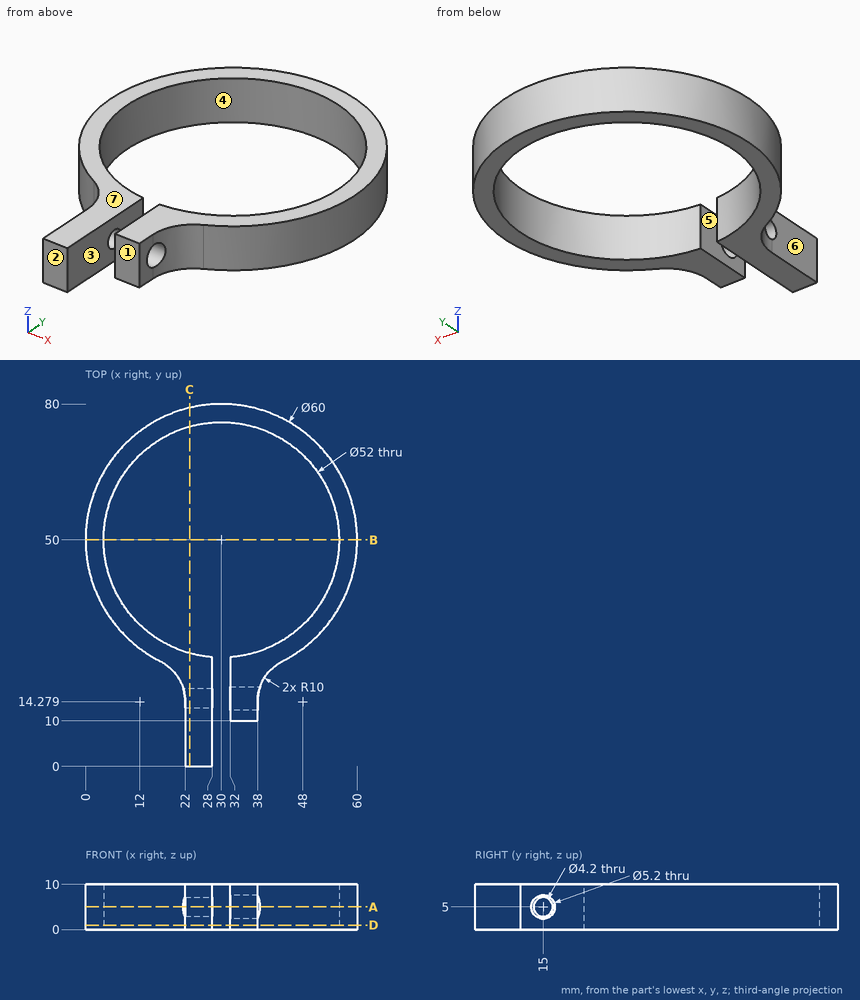
Check sheet for the drawn part. Datum: minimum x, y, z corner. Units: mm. A direction names the side the tool comes from. Coordinates: 2 decimals unless noted, no trailing zeros. Order: outer loops, then holes, each group sorted by start corner. A loop starts at its lowest first (then second) coordinate and runs counter-clockwise, first axis right, second up. Notation, with made-up numbers: (-20.5, -23.75) -> (18.5, -23.75) arc R28 cw to (18.5, 0.25) -> close; hole circle Ø8 at (29, -29). An arc over 180 degrees is marked (long way). Use a Markdown table: item, result. Add a question column.
1. Material ranges on L1, parallel to X at y = 13.5, z = 1.25; L2, parallel to Z at x = 25, y = 15; L3, parallel to X at y = 50, z = 4, recorded low to high.
2. Cross-section at C-C (x = 23). Enter the section's corners in (y, z), and give its area (3 significant figures).
3. Set-up check for the marked faces 1, 2 and 3: record each of +Z, -Z, +X, -X, +Y, -Y from which the full face is reachable in a straight line by a thin tool's end or side.
4. Cross-section at D-D (z = 1). Enter the section's corners in (x, y).
5. Cross-section at B-B (y = 50). Enter the section's corners in (x, z).
6. Go/stop test with flat-tipped pins: pin 1 Ø6 at (y, z) = (61.5, 9) entering from +X; pin 2 Ø2 at (x, z) = (50.5, 2.5) entering from -Y; pin 3 Ø4.5 at (y, z) = (13, 6) entering from +X; pin 4 Ø3 at (y, z) = (15, 5) entering from +X. Record where each tip stops, or that it passes through.
7. Cross-section at A-A (z = 5). Enter the section's corners in (x, y).
8. Mould release check, pull along X, two halves, no side actions. Record for the marked faces 4, 5, 6 and 7: pulls with the +X half, pulls with the -X half, needs draft (parallel to the pull), parting line crosses it, or undercut.
Filled sheet:
| question | item | result |
|---|---|---|
| 1 | L1 | 22 to 28, 32 to 38 |
| 1 | L2 | 0 to 2.9, 7.1 to 10 |
| 1 | L3 | 0 to 4, 56 to 60 |
| 2 | outline | (0, 0) -> (24.96, 0) -> (24.96, 10) -> (0, 10) -> close; (75.04, 0) -> (79.17, 0) -> (79.17, 10) -> (75.04, 10) -> close; hole circle Ø4.2 at (15, 5) |
| 2 | area | 277 mm2 |
| 3 | face 1 | +Z, -Z, +X, -Y |
| 3 | face 2 | +Z, -Z, +X, -X, -Y |
| 3 | face 3 | +Z, -Z, -Y |
| 4 | outline | (16.5, 23.21) arc R10 cw to (22, 14.28) -> (22, 0) -> (28, 0) -> (28, 24.08) arc R26 cw (long way) to (32, 24.08) -> (32, 10) -> (38, 10) -> (38, 14.28) arc R10 cw to (43.5, 23.21) arc R30 ccw (long way) to start |
| 5 | outline | (0, 0) -> (4, 0) -> (4, 10) -> (0, 10) -> close; (56, 0) -> (60, 0) -> (60, 10) -> (56, 10) -> close |
| 6 | pin 1 | x = 58.77 |
| 6 | pin 2 | y = 27.2 |
| 6 | pin 3 | x = 38.01 |
| 6 | pin 4 | through |
| 7 | outline | (16.5, 23.21) arc R10 cw to (21.59, 17.1) -> (28, 17.1) -> (28, 24.08) arc R26 cw (long way) to (32, 24.08) -> (32, 17.6) -> (38.57, 17.6) arc R10 cw to (43.5, 23.21) arc R30 ccw (long way) to start; (22, 0) -> (28, 0) -> (28, 12.9) -> (22, 12.9) -> close; (32, 10) -> (38, 10) -> (38, 12.4) -> (32, 12.4) -> close |
| 8 | face 4 | undercut |
| 8 | face 5 | undercut |
| 8 | face 6 | pulls with the -X half |
| 8 | face 7 | needs draft |
